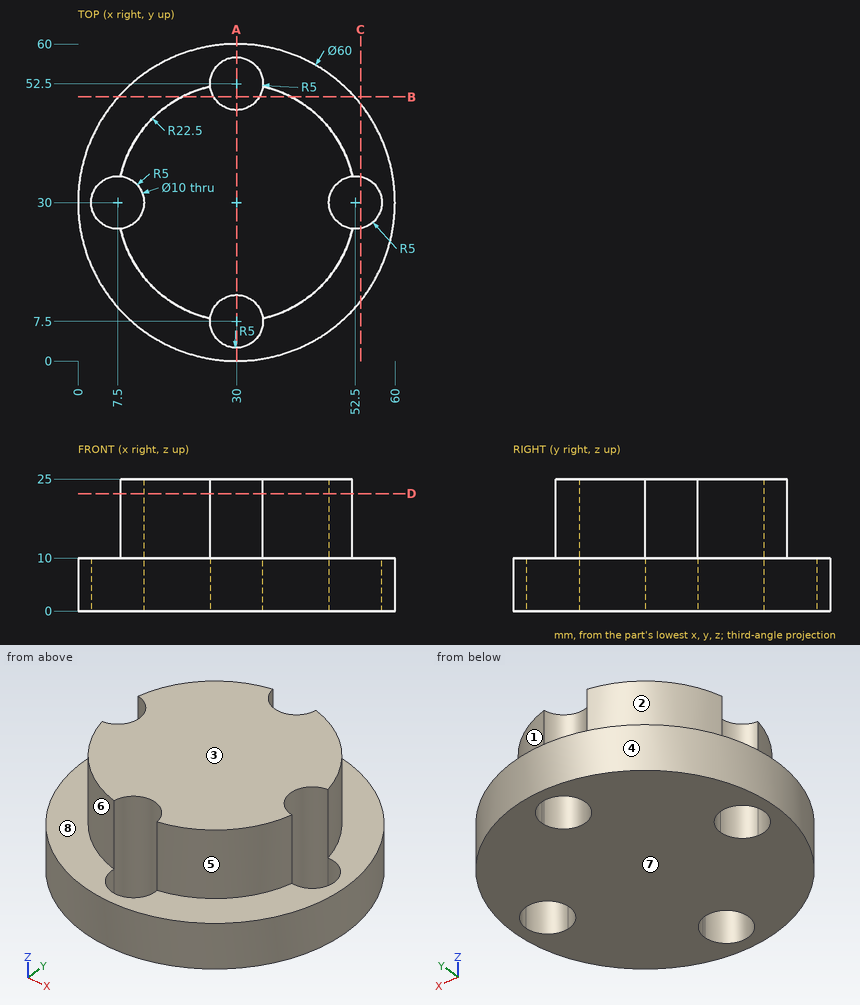
Verification items for this drawing (mm, ordinates from the low corner). A direction names the side the tool comes from. Give positions to 0.01 mm unless a question says otherwise; leave off trailing zeros. Write each loop counter-clockwise with the first axis right and the second up, starting at its lowest first coordinate (ties: lowest second). Pieces come first, ordered by that corner, then holes.
1) Go/stop test with flat-tipped pins: pin 1 Ø5 at (y, z) = (53, 19.5) entering from +X; pin 2 Ø2 at (x, z) = (19, 20) entering from +Y; pin 3 Ø2 at (y, z) = (49.5, 6.5) entering from -X. Record where each tip stops, or that it passes through.
Values follow:
pin 1: stops at x = 39.27
pin 2: stops at y = 50.16
pin 3: stops at x = 6.38
2) Cross-section at D-D (z = 22.25). Record the boundary of the cut face in (x, y).
Values follow:
outline: (8.06, 25.03) arc R22.5 ccw to (25.03, 8.06) arc R5 cw to (34.97, 8.06) arc R22.5 ccw to (51.94, 25.03) arc R5 cw to (51.94, 34.97) arc R22.5 ccw to (34.97, 51.94) arc R5 cw to (25.03, 51.94) arc R22.5 ccw to (8.06, 34.97) arc R5 cw to start
3) Cross-section at C-C (x = 53.5). Record the boundary of the cut face in (y, z).
Values follow:
outline: (11.35, 0) - (25.1, 0) - (25.1, 10) - (11.35, 10) - close; (34.9, 0) - (48.65, 0) - (48.65, 10) - (34.9, 10) - close
4) Cross-section at B-B (y = 50). Record the boundary of the cut face in (x, z), plus the area to 3 significant figures.
Values follow:
outline: (7.64, 0) - (25.67, 0) - (25.67, 25) - (19.69, 25) - (19.69, 10) - (7.64, 10) - close; (34.33, 0) - (52.36, 0) - (52.36, 10) - (40.31, 10) - (40.31, 25) - (34.33, 25) - close
area: 540 mm2
5) Cross-section at A-A (x = 30). Record the boundary of the cut face in (y, z).
Values follow:
outline: (0, 0) - (2.5, 0) - (2.5, 10) - (0, 10) - close; (12.5, 0) - (47.5, 0) - (47.5, 25) - (12.5, 25) - close; (57.5, 0) - (60, 0) - (60, 10) - (57.5, 10) - close
6) Release check for a two-part mould opening along X. For the marked faces 1, 2, 3 and 4 record: released by +X, released by -X, zero draft, split by the parting line, or undercut.
Values follow:
face 1: released by +X
face 2: released by -X
face 3: zero draft
face 4: split by the parting line
7) Set-up check for the marked faces 5, 6, 7 and 8: record each of +Z, -Z, +X, -X, +Y, -Y from which the full face is reachable in a straight line by a thin tool's end or side.
Values follow:
face 5: +Z, +X, -Y
face 6: +Z, -X, -Y
face 7: -Z, +X, -X, +Y, -Y
face 8: +Z
8) Thickness scan on line 1 (Z direction, x = 17, y = 56.5); line 2 (X direction, y = 33.5, z = 2.25); line 3 (X direction, y = 51, z = 9.25). Record the ranges inside material, lowest first.
Values follow:
line 1: z = 0 to 10
line 2: x = 0.2 to 3.93, 11.07 to 48.93, 56.07 to 59.8
line 3: x = 8.58 to 25.23, 34.77 to 51.42
